Autodesk Inventor part; units mm, degrees
ref_plane "YZ Plane" through (0, 0, 0) normal (1, 0, 0) x (0, 1, 0)
ref_plane "XZ Plane" through (0, 0, 0) normal (0, 1, 0) x (-1, 0, 0)
ref_plane "XY Plane" through (0, 0, 0) normal (0, 0, 1) x (1, 0, 0)
sketch "Sketch1" plane through (0, 0, 0) normal (0, 0, 1) x (1, 0, 0)
  line L0 (-6.9, 4.9) -> (6.9, 4.9)
  line L1 (6.9, 4.9) -> (6.9, -4.9)
  line L2 (6.9, -4.9) -> (-6.9, -4.9)
  line L3 (-6.9, -4.9) -> (-6.9, 4.9)
  circle A0 centre (0, 0) radius 1.925
  line L4 (-6.9, -1.5) -> (-11.9, -1.5)
  line L5 (-11.9, -1.5) -> (-11.9, 1.5)
  line L6 (-11.9, 1.5) -> (-6.9, 1.5)
  line L7 (-6.9, 1.5) -> (-6.9, -1.5)
  line L8 (6.9, -1.5) -> (11.9, -1.5)
  line L9 (11.9, -1.5) -> (11.9, 1.5)
  line L10 (11.9, 1.5) -> (6.9, 1.5)
  line L11 (6.9, 1.5) -> (6.9, -1.5)
  dimension "d0" = 13.8
  dimension "d1" = 9.8
  dimension "d2" = 6.9
  dimension "d3" = 4.9
  dimension "d6" = 3.85
  dimension "d7" = 3
  dimension "d8" = 1.5
  dimension "d9" = 5
  dimension "d10" = 5
extrude "Extrusion1" add sketch "Sketch1" along normal blind 2.3 contours L0 L1 L2 L3
extrude "Extrusion2" add sketch "Sketch1" along normal blind 1.5 contours L3 L4 L5 L6 | L10 L9 L8 L1
chamfer "Chamfer1" distance 1 angle 45 2 edges at (-11.9, 0, 1.5) (11.9, 0, 1.5)
sketch "Sketch2" plane through (0, 0, 1.5) normal (0, 0, 1) x (1, 0, 0)
  circle A0 centre (8.9, 0) radius 1
  line L0 (10.9, 1.5) -> (6.9, 1.5)
  line L1 (0, 0) -> (0.8425, 0) construction
  line L2 (6.9, -4.9) -> (6.9, 4.9)
  circle A1 centre (-8.9, 0) radius 1
  line L3 (-6.9, 4.9) -> (-6.9, -4.9)
  dimension "d17" = 2
  dimension "d19" = 2
  dimension "d20" = 2
  dimension "d21" = 2
extrude "Extrusion3" add sketch "Sketch2" along normal blind 1.5
sketch "Sketch3" plane through (0, 0, 0) normal (0, 1, 0) x (-1, 0, 0)
  line L0 (9.9, 3) -> (7.9, 3)
  circle A0 centre (8.9, 3) radius 1.15
  line L1 (7.9, 1.5) -> (7.9, 3)
  line L2 (9.9, 1.5) -> (9.9, 3)
  line L3 (-7.9, 3) -> (-9.9, 3)
  circle A1 centre (-8.9, 3) radius 1.15
  line L4 (-9.9, 1.5) -> (-9.9, 3)
  line L5 (9.9, 3) -> (10.05, 3)
  line L6 (7.9, 3) -> (7.75, 3)
  line L7 (-7.75, 3) -> (-10.05, 3)
  point P0 (0, 0)
  dimension "d24" = 0.15
  dimension "d25" = 0.15
revolve "Revolution1" add sketch "Sketch3" angle 360 about axis through (-9.9, 0, 3) along (-1, 0, 0) contours L0 L6 A0 L5 | L3 L7 A1
fillet "Fillet1" radius 0.5 4 edges at (-6.9, -4.9, 1.15) (-6.9, 4.9, 1.15) (6.9, 4.9, 1.15) (6.9, -4.9, 1.15)
equation "\"d10\" = d9"
equation "\"d20\" = d17"
equation "\"d21\" = d19"
properties part number "motor_cover_3DPrint"
Input: part model. Units: mm. Frame: model coordinates. A direction names the side the tool comes from. Give positions to 0.01 mm unless a question says otherwise; leave off trailing zeros. Write each loop counter-clockwise with the first axis right and the second up, starting at its lowest first coordinate (ties: lowest second). Pieces come first, ordered by that corner, then holes. Notation, with made-up numbers: (6.5, 50.25) -> (15.5, 50.25) arc R22 cw to (15.5, 89.25) -> close; hole circle Ø1 at (9, -14). An arc over 180 degrees is marked (long way). Use one line per item in the form item = value. Start each with the question number.
1) Pin query (flat end, axial travel): pin 1 (0.7 mm diameter, centred on y = 0, z = 1, fed in from +X); pin 2 (0.8 mm diameter, centred on x = -10, z = 1, fed in from +Y); pin 3 (2 mm diameter, centred on x = -9.5, z = 3.5, fed in from -Y); pin 4 (1 mm diameter, centred on y = 3.5, z = 3.5, fed in from +X). Return the tip coordinate at first contact, or that it passes through.
2) Draft query along X for faces 5 (the flat face through (11.4, 0, 1)), 6 (the flat face through (-11.4, 0, 1)), 7 (the flat face through (-8, 1, 1.5)). Return one class per face: pulls with the +X half, pulls with the -X half, needs draft (parallel to the pull), parting line crosses it, or undercut.
3) Section query C-C on x = 9.5. Return the cut outline in (y, z).
4) Ray query, probe 1 along Y at (x, z) = (0, 0.8) (3 decimals); probe 2 along X at (y, z) = (0, 3.05); probe 3 along Z at (x, y) = (5.5, 0.25). Return the intervals inside material, ascending. Write a range as from..to.
5) Set-up query: faces 1 (the flat face through (9, 1.5, 1)), 2 (the flat face through (9, -1.5, 1)), 3 (the flat face through (-9, -1.5, 1)), 4 (the cylindrical face through (7.9, 0, 2)). Return all of +Z, -Z, +X, -X, +Y, -Y with unobstructed straight access to the full face (end or side cutting, diameter ignored); none if empty.
6) Section query D-D on y = -3. Return the cut outline in (x, z), then the cut area to 3 significant figures.
7) Section query B-B on z = 1.2. Return the cut outline in (x, y) (3 decimals).
8) Section query A-A on x = 0. Return the cut outline in (y, z) (3 decimals), then the cut area to 3 significant figures.
Outcome:
q1.pin_1 = 11.75
q1.pin_2 = 1.5
q1.pin_3 = -1.15
q1.pin_4 = through
q2.face_5 = pulls with the +X half
q2.face_6 = pulls with the -X half
q2.face_7 = undercut
q3.outline = (-1.5, 0) -> (1.5, 0) -> (1.5, 1.5) -> (0.8, 1.5) -> (0.8, 2.43) arc R0.98 ccw (long way) to (-0.8, 2.43) -> (-0.8, 1.5) -> (-1.5, 1.5) -> close
q4.probe_1 = -4.9..-1.925, 1.925..4.9
q4.probe_2 = -10.05..-7.75, 7.75..10.05
q4.probe_3 = 0..2.3
q5.face_1 = +Z, -Z, +X, +Y
q5.face_2 = +Z, -Z, +X, -Y
q5.face_3 = +Z, -Z, -X, -Y
q5.face_4 = none
q6.outline = (-6.9, 0) -> (6.9, 0) -> (6.9, 2.3) -> (-6.9, 2.3) -> close
q6.area = 31.7 mm^2
q7.outline = (-11.2, -1.5) -> (-6.9, -1.5) -> (-6.9, -4.4) arc R0.5 ccw to (-6.4, -4.9) -> (6.4, -4.9) arc R0.5 ccw to (6.9, -4.4) -> (6.9, -1.5) -> (11.2, -1.5) -> (11.2, 1.5) -> (6.9, 1.5) -> (6.9, 4.4) arc R0.5 ccw to (6.4, 4.9) -> (-6.4, 4.9) arc R0.5 ccw to (-6.9, 4.4) -> (-6.9, 1.5) -> (-11.2, 1.5) -> close; hole circle Ø3.85 at (0, 0)
q8.outline = (-4.9, 0) -> (-1.925, 0) -> (-1.925, 2.3) -> (-4.9, 2.3) -> close; (1.925, 0) -> (4.9, 0) -> (4.9, 2.3) -> (1.925, 2.3) -> close
q8.area = 13.7 mm^2
